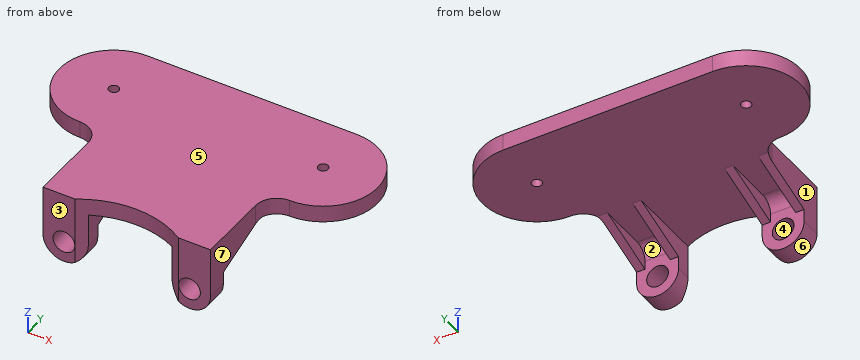
from build123d import *

# Parameters (mm, degrees)
EXTRUDE_1_OUTLINE_R             = 1.2
EXTRUDE_1_DEPTH                 = 4
SKETCH_2_R                      = 2.6
EXTRUDE_2_DEPTH                 = 5
CUT_EXTRUDE_1_REACH             = 55.603
CUT_EXTRUDE_1_DIRECTION_2_DEPTH = 54.602705156
EXTRUDE_4_DEPTH                 = 2
EXTRUDE_5_DEPTH                 = 2
FILLET_1_R                      = 3
FILLET_2_R                      = 5


# Read off the part's stored shape, not the designer's step: 凸台-拉伸1
with BuildPart() as part:
    # 凸台-拉伸1 outline → 凸台-拉伸1 (new body)
    with BuildSketch(Plane.XY):
        with BuildLine():
            ThreePointArc((-25, 13), (-38, 0), (-25, -13))
            Line((-25, -13), (-20, -13))
            Line((-20, -13), (-20, -35.5))
            Line((-20, -35.5), (20, -35.5))
            Line((20, -35.5), (20, -13))
            Line((20, -13), (25, -13))
            ThreePointArc((25, -13), (38, 0), (25, 13))
            Line((25, 13), (-25, 13))
        make_face()
        with Locations((-25, 0)):
            Circle(EXTRUDE_1_OUTLINE_R, mode=Mode.SUBTRACT)
        with Locations((25, 0)):
            Circle(EXTRUDE_1_OUTLINE_R, mode=Mode.SUBTRACT)
    extrude(amount=EXTRUDE_1_DEPTH)

    # 草图2 → 凸台-拉伸2 (add)
    # profile 1 of 2: a face of its own
    with BuildSketch(Plane.XZ.offset(35.5)):
        with BuildLine():
            Line((-20, -8), (-20, 0))
            Line((-20, 0), (-20, 4))
            Line((-20, 4), (-10, 4))
            Line((-10, 4), (-10, 0))
            Line((-10, 0), (-10, -8))
            ThreePointArc((-10, -8), (-15, -13), (-20, -8))
        make_face()
        with Locations(Location((-15, -8, 0), (0, 0, 270))):
            Circle(SKETCH_2_R, mode=Mode.SUBTRACT)
    # profile 2 of 2: a face of its own
    with BuildSketch(Plane.XZ.offset(35.5)):
        with BuildLine():
            Line((20, 0), (20, 4))
            Line((20, 4), (10, 4))
            Line((10, 4), (10, 0))
            Line((10, 0), (10, -8))
            ThreePointArc((10, -8), (15, -13), (20, -8))
            Line((20, -8), (20, 0))
        make_face()
        with Locations(Location((15, -8, 0), (0, 0, 270))):
            Circle(SKETCH_2_R, mode=Mode.SUBTRACT)
    extrude(amount=-EXTRUDE_2_DEPTH)

    # 草图3 → 切除-拉伸1 (cut, up to next)
    with BuildSketch(Plane(origin=(0, 0, 0), x_dir=(-1, 0, 0), z_dir=(0, 0, -1)), mode=Mode.PRIVATE) as cut_extrude_1_sk1:
        with BuildLine():
            Line((-12.329740468, -35.5), (12.329740468, -35.5))
            ThreePointArc((12.329740468, -35.5), (0, -31.85), (-12.329740468, -35.5))
        make_face()
    cut_extrude_1_tool1 = extrude(cut_extrude_1_sk1.sketch, amount=-CUT_EXTRUDE_1_REACH, mode=Mode.PRIVATE) & part.part
    add(cut_extrude_1_tool1.solids().sort_by_distance((0, -34.029422, 0))[0], mode=Mode.SUBTRACT)

    # 草图3 → 切除-拉伸1 direction 2 (cut)
    with BuildSketch(Plane(origin=(0, 0, 0), x_dir=(-1, 0, 0), z_dir=(0, 0, -1))):
        with BuildLine():
            Line((-12.329740468, -35.5), (12.329740468, -35.5))
            ThreePointArc((12.329740468, -35.5), (0, -31.85), (-12.329740468, -35.5))
        make_face()
    extrude(amount=CUT_EXTRUDE_1_DIRECTION_2_DEPTH, mode=Mode.SUBTRACT)

    # 草图5 → 凸台-拉伸4 (add)
    with BuildSketch(Plane(origin=(20, 0, 0), x_dir=(0, 0, -1), z_dir=(1, 0, 0))):
        Polygon((0, -16), (5, -30.5), (0, -30.5), align=None)
    extrude_4 = extrude(amount=-EXTRUDE_4_DEPTH)

    # 草图6 → 凸台-拉伸5 (add)
    with BuildSketch(Plane.ZY.offset(-10)):
        Polygon((-5, -30.5), (0, -16), (0, -30.5), align=None)
    extrude_5 = extrude(amount=-EXTRUDE_5_DEPTH)

    # 镜向1: 凸台-拉伸4, 凸台-拉伸5 across plane
    add(extrude_4.mirror(Plane(origin=(0, 0, 0), x_dir=(0, 0, 1), z_dir=(1, 0, 0))))
    add(extrude_5.mirror(Plane(origin=(0, 0, 0), x_dir=(0, 0, 1), z_dir=(1, 0, 0))))

    # 圆角1
    fillet_1_edges = [part.edges().sort_by_distance(p)[0] for p in [
        (15, -30.5, 0),
        (-15, -30.5, 0),
    ]]
    fillet(fillet_1_edges, radius=FILLET_1_R)

    # 圆角2
    fillet_2_edges = [part.edges().sort_by_distance(p)[0] for p in [
        (-20, -13, 2),
        (20, -13, 2),
    ]]
    fillet(fillet_2_edges, radius=FILLET_2_R - 0.0001)  # a hair under: the kernel refuses the full size


solid = part.part
Work out the finished part from the listing and answer in its coordinate system (mm). Face numbers are marked on the shaded views. A direction names the side the tool comes from. Give positions to 0.01 mm unless a question says otherwise; leave off trailing zeros. Loops run counter-clockwise (first coordinate to the right, second up) from the corner with the lowest first, then second, coordinate; pieces in that order, holes last. Notation, with made-up numbers: (27, 85.25) -> (70, 85.25) arc R15 cw to (70, 104.25) -> close; hole circle Ø3 at (80, 75). An arc over 180 degrees is marked (long way). Use a Markdown table: item, result. Add a question column.
1. Section B-B on y = 0 is taken. Determine the outline of the cut face in (x, z).
2. Section D-D on z = 0.75 is taken. State how many separate pieces and enclosed holes the cut face has, and give its area (3 significant figures).
3. Find the intervals of material crossed by probe 1 along X at (y, z) = (-31.9, -8); probe 2 along X at (y, z) = (-18, -0.5); probe 3 along Y at (x, z) = (-25, 3), in increasing order.
4. Section C-C on z = -4.25 is taken. Determine the outline of the cut face in (x, y) (3 decimals), and give its area (3 significant figures).
5. For the marked faces 1, 2 and 3, determine the directions among +Z, -Z, +X, -X, +Y, -Y from which every point of the face is accessible in a straight line to the end or side of a thin tool.
6. Determine the mould class of the marked faces 4, 5, 6 and 7 for opening direction X: released by +X, released by -X, zero draft, split by the parting line, or undercut.
7. Flat-ended cylindrical pins translate along their axes: pin 1 Ø3.5 at (y, z) = (-25, -3) entering from -X; pin 2 Ø1 at (y, z) = (3, 2) entering from +X; pin 3 Ø5.5 at (y, z) = (-24.5, -1.5) entering from +X. Find the tip coordinate at first contact, or state that the pin passes through.
8. Section A-A on x = -15 is taken. Determine the outline of the cut face in (y, z), and give its area (3 significant figures).
Results below:
| question | item | result |
|---|---|---|
| 1 | outline | (-38, 0) -> (-26.2, 0) -> (-26.2, 4) -> (-38, 4) -> close; (-23.8, 0) -> (23.8, 0) -> (23.8, 4) -> (-23.8, 4) -> close; (26.2, 0) -> (38, 0) -> (38, 4) -> (26.2, 4) -> close |
| 2 | separate pieces | 1 |
| 2 | enclosed holes | 2 |
| 2 | area | 2,670 mm^2 |
| 3 | probe 1 | x = -20 to -17.6, -12.4 to -10, 10 to 12.4, 17.6 to 20 |
| 3 | probe 2 | x = -20 to -18, -12 to -10, 10 to 12, 18 to 20 |
| 3 | probe 3 | y = -13 to -1.2, 1.2 to 13 |
| 4 | outline | (-20, -35.5) -> (-12.33, -35.5) arc R22.65 cw to (-10, -34.177) -> (-10, -28.325) -> (-12, -28.325) -> (-12, -30.5) -> (-18, -30.5) -> (-18, -28.325) -> (-20, -28.325) -> close; (10, -34.177) arc R22.65 cw to (12.33, -35.5) -> (20, -35.5) -> (20, -28.325) -> (18, -28.325) -> (18, -30.5) -> (12, -30.5) -> (12, -28.325) -> (10, -28.325) -> close |
| 4 | area | 114 mm^2 |
| 5 | face 1 | +Z, -Z, -X, -Y |
| 5 | face 2 | -Z, +Y |
| 5 | face 3 | +Z, -Z, +X, -X, -Y |
| 6 | face 4 | undercut |
| 6 | face 5 | zero draft |
| 6 | face 6 | undercut |
| 6 | face 7 | released by +X |
| 7 | pin 1 | stops at x = -20 |
| 7 | pin 2 | stops at x = 37.76 |
| 7 | pin 3 | stops at x = 20 |
| 8 | outline | (-35.5, -13) -> (-30.5, -13) -> (-30.5, -10.6) -> (-35.5, -10.6) -> close; (-35.5, -5.4) -> (-30.5, -5.4) -> (-30.5, -3) arc R3 cw to (-27.5, 0) -> (13, 0) -> (13, 4) -> (-35.5, 4) -> close |
| 8 | area | 235 mm^2 |
